Geometry check sheet. Reference: the model listing, model coordinates, mm. A direction names the side the tool comes from. Coordinates: 2 decimals unless noted, no trailing zeros. Order: outer loops, then holes, each group sorted by start corner. A loop starts at its lowest first (then second) coordinate and runs counter-clockwise, first axis right, second up. Notation, with made-up numbers: M -40,18.25 L -20,18.25 A8 ccw -20,22.25 Z; hole C 51,76 d5. An arc over 180 degrees is marked long. One line per item, written item: value. Start each with the question number.
1) Go/stop test with flat-tipped pins: P1, Ø1.5, axis at y = 11, z = 52, coming from the -X side; P2, Ø2, axis at x = 26, y = 4.5, coming from the +Z side. Record where each tip stops, or that it passes through.
2) Sectioned sample at C-C, the plane z = 65. Enter the section's corners in (x, y).
3) Access from +Z, -Z, +X, -X, +Y, -Y to the whole of each face (thin tool, end or side, straight path). Record for faces 1 (the flat face through (0, -20, 49)), 2 (the flat face through (-16, 15, 49)).
4) Sectioned sample at A-A, the plane y = -6. Enter the section's corners in (x, z), then the cut area to 3 significant figures.
5) Draft check along X on faces 3 (the flat face through (28.1, 13.2, 6.1)), 4 (the flat face through (16, 15, 49)), 5 (the flat face through (-28.9, -16.2, 49.4)). Enter one of: pulls with the +X half, pulls with the -X half, needs draft (parallel to the pull), parting line crosses it, or undercut.
6) Thickness scan on L1, parallel to X at y = 10, z = 65; L2, parallel to X at y = -14, z = 18.5; L3, parallel to Y at x = 2, z = 65. Record the ranges inside material, lowest first. Write a range as from..to.
7) Sectioned sample at B-B, the plane z = 41.5. Enter the section's corners in (x, y).
8) Sectioned sample at D-D, the plane x = 27.5. Enter the section's corners in (y, z).
```python
from build123d import *

# Parameters (mm, degrees)
F0_W          = 5
F0_H          = 30
F2_DEPTH      = 90
F0_W_2        = 70
F0_H_2        = 40
F3_DEPTH      = 90
F0_W_3        = 27.5
F4_DEPTH      = 10
F1_R          = 7.5
F5_DEPTH      = 15
F5_DEPTH_BACK = 25
F6_SIZE       = 9.9


with BuildPart() as f2:
    # F0 (on Top) → F2 (new body)
    with BuildSketch(Plane.XY):
        Rectangle(F0_W, F0_H)
    extrude(amount=F2_DEPTH)

    # F0 (on Top) → F3 (join)
    with BuildSketch(Plane.XY):
        Rectangle(F0_W_2, F0_H_2)
        Polygon((-30, -15), (-30, 15), (-2.5, 15), (2.5, 15), (30, 15), (30, -15), (2.5, -15), (-2.5, -15), align=None, mode=Mode.SUBTRACT)
    extrude(amount=F3_DEPTH)

    # F0 (on Top) → F4 (join)
    with BuildSketch(Plane.XY):
        with Locations((-16.25, 0)):
            Rectangle(F0_W_3, F0_H)
        with Locations((16.25, 0)):
            Rectangle(F0_W_3, F0_H)
    extrude(amount=F4_DEPTH)

    # F1 (on Right) → F5 (cut, two sides)
    with BuildSketch(Plane.YZ) as f5_sk:
        with Locations((0, 65)):
            Circle(F1_R)
    extrude(amount=F5_DEPTH, mode=Mode.SUBTRACT)
    extrude(f5_sk.sketch, amount=-F5_DEPTH_BACK, mode=Mode.SUBTRACT)

    # F6
    f6_edges = [f2.edges().sort_by_distance(p)[0] for p in [
        (35, -20, 45),
        (35, 20, 45),
        (-35, 20, 45),
        (-35, -20, 45),
        (0, 20, 0),
        (35, 0, 0),
        (0, -20, 0),
        (-35, 0, 0),
    ]]
    chamfer(f6_edges, length=F6_SIZE)


solid = f2.part
```
Final values:
1. P1: stops at x = -34.85
1. P2: stops at z = 10
2. outline: M -35,-10.1 L -25.1,-20 L 25.1,-20 L 35,-10.1 L 35,10.1 L 25.1,20 L -25.1,20 L -35,10.1 Z; hole M -30,-15 L -2.5,-15 L -2.5,-7.5 L 2.5,-7.5 L 2.5,-15 L 30,-15 L 30,15 L 2.5,15 L 2.5,7.5 L -2.5,7.5 L -2.5,15 L -30,15 Z
3. face 1: +Z, -Z, +X, -X, -Y
3. face 2: +Z
4. outline: M -35,9.9 L -25.1,0 L 25.1,0 L 35,9.9 L 35,90 L 30,90 L 30,10 L 2.5,10 L 2.5,60.5 L -2.5,60.5 L -2.5,10 L -30,10 L -30,90 L -35,90 Z; M -2.5,69.5 L 2.5,69.5 L 2.5,90 L -2.5,90 Z
4. area: 1,760 mm^2
5. face 3: pulls with the +X half
5. face 4: undercut
5. face 5: pulls with the -X half
6. L1: x = -35..-30, -2.5..2.5, 30..35
6. L2: x = -31.1..-30, -2.5..2.5, 30..31.1
6. L3: y = -20..-7.5, 7.5..20
7. outline: M -35,-10.1 L -25.1,-20 L 25.1,-20 L 35,-10.1 L 35,10.1 L 25.1,20 L -25.1,20 L -35,10.1 Z; hole M -30,-15 L -2.5,-15 L -2.5,15 L -30,15 Z; hole M 2.5,-15 L 30,-15 L 30,15 L 2.5,15 Z
8. outline: M -17.6,9.9 L -10.1,2.4 L 10.1,2.4 L 17.6,9.9 L 17.6,90 L 15,90 L 15,10 L -15,10 L -15,90 L -17.6,90 Z
